The model under review builds one solid part; all positions refer to its coordinate system, in mm. A direction names the side the tool comes from. Round coordinates to 2 decimals unless told otherwise and drop trailing zeros. Loops run counter-clockwise (first coordinate to the right, second up) from the corner with the lowest first, then second, coordinate; pieces in that order, holes last. Notation, with made-up numbers: M -26.5,32.5 L 22.5,32.5 A32 ccw 22.5,60.5 Z; hole C -19.5,-17.75 d9. An arc over 180 degrees is marked long. Use a Markdown table: item, result. Add a question column.
```python
from build123d import *

# Parameters (mm, degrees)
X_ANGLE_LENTH_DEPTH             = 1574.8
X_ANGLE_LENTH_2_DEPTH           = 1574.8
X_ANGLE_LENTH_3_DEPTH           = 1574.8
X_ANGLE_LENTH_4_DEPTH           = 1574.8
Y_ANGLE_LENTH_DEPTH             = 209.55
Z_START                         = -457.2
Z_ANGLE_LENTH_DEPTH             = 914.4
SKETCH16_R                      = 4.7625
WHEEL_MOUNT_LOC_HOLES_DEPTH     = 210.55
SKETCH17_W                      = 50.8
SKETCH17_H                      = 38.1
FRONT_CONTROL_ARM_CUTOUTS_DEPTH = 1017
SKETCH19_R                      = 4
CUT_EXTRUDE1_DEPTH              = 7.35


with BuildPart() as part:
    # Sketch5 → X Angle Lenth (new body)
    with BuildSketch(Plane(origin=(0, 0, 0), x_dir=(0, 0, -1), z_dir=(1, 0, 0))):
        Polygon((-508, -304.8), (-508, -254), (-501.65, -254), (-501.65, -298.45), (-457.2, -298.45), (-457.2, -304.8), align=None)
    extrude(amount=X_ANGLE_LENTH_DEPTH)



with BuildPart() as body_2:
    # Sketch5 → X Angle Lenth 2 (new body)
    with BuildSketch(Plane(origin=(0, 0, 0), x_dir=(0, 0, -1), z_dir=(1, 0, 0))):
        Polygon((501.65, -254), (508, -254), (508, -304.8), (457.2, -304.8), (457.2, -298.45), (501.65, -298.45), align=None)
    extrude(amount=X_ANGLE_LENTH_2_DEPTH)


with BuildPart() as body_3:
    # Sketch5 → X Angle Lenth 3 (new body)
    with BuildSketch(Plane(origin=(0, 0, 0), x_dir=(0, 0, -1), z_dir=(1, 0, 0))):
        Polygon((508, -95.25), (508, -146.05), (501.65, -146.05), (501.65, -101.6), (457.2, -101.6), (457.2, -95.25), align=None)
    extrude(amount=X_ANGLE_LENTH_3_DEPTH)


with BuildPart() as body_4:
    # Sketch5 → X Angle Lenth 4 (new body)
    with BuildSketch(Plane(origin=(0, 0, 0), x_dir=(0, 0, -1), z_dir=(1, 0, 0))):
        Polygon((-501.65, -146.05), (-508, -146.05), (-508, -95.25), (-457.2, -95.25), (-457.2, -101.6), (-501.65, -101.6), align=None)
    extrude(amount=X_ANGLE_LENTH_4_DEPTH)


with BuildPart() as part_1:
    add(part.part)

    add(body_2.part)  # Y Angle Lenth merges body 2

    add(body_3.part)  # Y Angle Lenth merges body 3

    add(body_4.part)  # Y Angle Lenth merges body 4
    # Sketch6 → Y Angle Lenth (add)
    with BuildSketch(Plane.XZ.offset(304.8)):
        Polygon((1574.8, -508), (1524, -508), (1524, -501.65), (1568.45, -501.65), (1568.45, -457.2), (1574.8, -457.2), align=None)
        Polygon((1524, 501.65), (1524, 508), (1574.8, 508), (1574.8, 457.2), (1568.45, 457.2), (1568.45, 501.65), align=None)
        Polygon((0, 508), (50.8, 508), (50.8, 501.65), (6.35, 501.65), (6.35, 457.2), (0, 457.2), align=None)
        Polygon((50.8, -501.65), (50.8, -508), (0, -508), (0, -457.2), (6.35, -457.2), (6.35, -501.65), align=None)
    extrude(amount=-Y_ANGLE_LENTH_DEPTH)

    # Sketch15 → Z Angle Lenth (add)
    with BuildSketch(Plane.XY.offset(Z_START)):
        Polygon((0, -254), (0, -304.8), (50.8, -304.8), (50.8, -298.45), (6.35, -298.45), (6.35, -254), align=None)
        Polygon((1568.45, -254), (1574.8, -254), (1574.8, -304.8), (1524, -304.8), (1524, -298.45), (1568.45, -298.45), align=None)
        Polygon((1574.8, -146.05), (1574.8, -95.25), (1524, -95.25), (1524, -101.6), (1568.45, -101.6), (1568.45, -146.05), align=None)
        Polygon((6.35, -146.05), (0, -146.05), (0, -95.25), (50.8, -95.25), (50.8, -101.6), (6.35, -101.6), align=None)
    extrude(amount=Z_ANGLE_LENTH_DEPTH)

    # Sketch16 → Wheel Mount LOC Holes (cut, through all)
    with BuildSketch(Plane(origin=(0, -95.25, 0), x_dir=(1, 0, 0), z_dir=(0, 1, 0))):
        with Locations((1409.7, 482.6)):
            Circle(SKETCH16_R)
        with Locations((1003.3, 482.6)):
            Circle(SKETCH16_R)
        with Locations((584.2, 482.6)):
            Circle(SKETCH16_R)
        with Locations((177.8, 482.6)):
            Circle(SKETCH16_R)
        with Locations((177.8, -482.6)):
            Circle(SKETCH16_R)
        with Locations((584.2, -482.6)):
            Circle(SKETCH16_R)
        with Locations((1003.3, -482.6)):
            Circle(SKETCH16_R)
        with Locations((1409.7, -482.6)):
            Circle(SKETCH16_R)
        with Locations((1054.1, 482.6)):
            Circle(SKETCH16_R)
        with Locations((1460.5, 482.6)):
            Circle(SKETCH16_R)
        with Locations((1460.5, -482.6)):
            Circle(SKETCH16_R)
        with Locations((1054.1, -482.6)):
            Circle(SKETCH16_R)
    extrude(amount=-WHEEL_MOUNT_LOC_HOLES_DEPTH, mode=Mode.SUBTRACT)

    # Sketch17 → Front Control Arm Cutouts (cut, through all)
    with BuildSketch(Plane.XY.offset(508)):
        with Locations((177.8, -254)):
            Rectangle(SKETCH17_W, SKETCH17_H)
        with Locations((584.2, -254)):
            Rectangle(SKETCH17_W, SKETCH17_H)
    extrude(amount=-FRONT_CONTROL_ARM_CUTOUTS_DEPTH, mode=Mode.SUBTRACT)

    # Sketch19 → Cut-Extrude1 (cut, through all)
    with BuildSketch(Plane(origin=(0, -298.45, 0), x_dir=(1, 0, 0), z_dir=(0, 1, 0))):
        with Locations((736.6, -469.9)):
            Circle(SKETCH19_R)
        with Locations((772.6, -469.9)):
            Circle(SKETCH19_R)
    extrude(amount=-CUT_EXTRUDE1_DEPTH, mode=Mode.SUBTRACT)


solid = part_1.part
```
(1) To check wall thickness, follow probe 1 along Z at (x, y) = (177.8, -301.25); probe 2 along Z at (x, y) = (736, -266.5); probe 3 along X at (y, z) = (-296, 36). State the ranges of each line that lie inside material, in increasing order.
(2) Consider section A-A, the plane y = -188. Give the boundary of the cut face in (x, z), then the cut area to 3 significant figures.
(3) Consider section B-B, the plane z = 165. Give the boundary of the cut face in (x, y).
(4) Draft analysis for pull direction Z (two halves, no side actions). For faces 1 (the face through (776, -132, 508)), 2 (the face through (1574.8, -132, 7)), 3 (the face through (6.35, -136, -7)), 4 (the face through (776, -133, 501.65)), state which applies: released by +Z, released by -Z, zero draft, split by the parting line, or undercut.
(5) For faces 5 (the face through (784, -95.25, 492)), 6 (the face through (784, -101.6, -485)), list the 3-axis set-ups (+Z, -Z, +X, -X, +Y, -Y) from which the entire face can be reached by the end or side of a thin tool; tool diameter is ignored.
(6) Insertion check: pin 1 Ø3 at (y, z) = (-263, -503.5) entering from -X. The pin has a flat end and moves straight along its axis. Give the tip position at first contact, or say it passes through.
Found:
| question | item | result |
|---|---|---|
| 1 | probe 1 | z = -508 to -487.36, -477.84 to -457.2, 457.2 to 477.84, 487.36 to 508 |
| 1 | probe 2 | z = -508 to -501.65, 501.65 to 508 |
| 1 | probe 3 | x = 0 to 6.35, 1568.45 to 1574.8 |
| 2 | outline | M 0,-508 L 50.8,-508 L 50.8,-501.65 L 6.35,-501.65 L 6.35,-457.2 L 0,-457.2 Z; M 0,457.2 L 6.35,457.2 L 6.35,501.65 L 50.8,501.65 L 50.8,508 L 0,508 Z; M 1524,-508 L 1574.8,-508 L 1574.8,-457.2 L 1568.45,-457.2 L 1568.45,-501.65 L 1524,-501.65 Z; M 1524,501.65 L 1568.45,501.65 L 1568.45,457.2 L 1574.8,457.2 L 1574.8,508 L 1524,508 Z |
| 2 | area | 2,420 mm^2 |
| 3 | outline | M 0,-304.8 L 50.8,-304.8 L 50.8,-298.45 L 6.35,-298.45 L 6.35,-254 L 0,-254 Z; M 0,-146.05 L 6.35,-146.05 L 6.35,-101.6 L 50.8,-101.6 L 50.8,-95.25 L 0,-95.25 Z; M 1524,-304.8 L 1574.8,-304.8 L 1574.8,-254 L 1568.45,-254 L 1568.45,-298.45 L 1524,-298.45 Z; M 1524,-101.6 L 1568.45,-101.6 L 1568.45,-146.05 L 1574.8,-146.05 L 1574.8,-95.25 L 1524,-95.25 Z |
| 4 | face 1 | released by +Z |
| 4 | face 2 | zero draft |
| 4 | face 3 | undercut |
| 4 | face 4 | undercut |
| 5 | face 5 | +Z, -Z, +X, -X, +Y |
| 5 | face 6 | none |
| 6 | pin 1 | stops at x = 0 |
